```python
from build123d import *

# Parameters (mm, degrees)
SKETCH1_R           = 1.5
SKETCH1_R_2         = 1.35
SKETCH1_R_3         = 1.3
BOSS_EXTRUDE1_DEPTH = 3
BOSS_EXTRUDE2_START = 2
SKETCH2_W           = 64
SKETCH2_H           = 44
SKETCH2_R           = 1.3
BOSS_EXTRUDE2_DEPTH = 2
SKETCH3_W           = 64
SKETCH3_H           = 44
SKETCH3_W_2         = 60
SKETCH3_H_2         = 40
BOSS_EXTRUDE3_DEPTH = 12
SKETCH4_W           = 61
SKETCH4_H           = 41
SKETCH4_W_2         = 60
SKETCH4_H_2         = 40
CUT_EXTRUDE1_DEPTH  = 9
SKETCH5_R           = 3
CUT_EXTRUDE2_DEPTH  = 9
CUT_EXTRUDE3_START  = -9
CUT_EXTRUDE3_DEPTH  = 9
SKETCH7_W           = 66
SKETCH7_H           = 46
SKETCH7_W_2         = 64
SKETCH7_H_2         = 44
BOSS_EXTRUDE4_DEPTH = 14
SKETCH8_W           = 66
SKETCH8_H           = 46
BOSS_EXTRUDE5_DEPTH = 2
SKETCH9_R           = 6
SKETCH9_R_2         = 1.5
BOSS_EXTRUDE7_DEPTH = 4
FILLET1_R           = 5
FILLET2_R           = 2


with BuildPart() as part:
    # Sketch1 → Boss-Extrude1 (new body)
    # profile 1 of 12: a face of its own
    with BuildSketch(Plane.XY):
        with BuildLine():
            Line((-25.901923789, 20), (-28.5, 20))
            ThreePointArc((-28.5, 20), (-27.439339828, 19.560660172), (-27, 18.5))
            ThreePointArc((-27, 18.5), (-28.5, 17), (-30, 18.5))
            Line((-30, 18.5), (-30, 15.901923789))
            ThreePointArc((-30, 15.901923789), (-27, 15.901923789), (-25.5, 18.5))
            ThreePointArc((-25.5, 18.5), (-25.602222521, 19.276457135), (-25.901923789, 20))
        make_face()
    # profile 2 of 12: a face of its own
    with BuildSketch(Plane.XY):
        with BuildLine():
            Line((28.5, 20), (25.901923789, 20))
            ThreePointArc((25.901923789, 20), (26.378679656, 16.378679656), (30, 15.901923789))
            Line((30, 15.901923789), (30, 18.5))
            ThreePointArc((30, 18.5), (27.439339828, 17.439339828), (28.5, 20))
        make_face()
    # profile 3 of 12: a face of its own
    with BuildSketch(Plane.XY):
        with BuildLine():
            Line((30, -18.5), (30, -15.901923789))
            ThreePointArc((30, -15.901923789), (26.378679656, -16.378679656), (25.901923789, -20))
            Line((25.901923789, -20), (28.5, -20))
            ThreePointArc((28.5, -20), (27.439339828, -17.439339828), (30, -18.5))
        make_face()
    # profile 4 of 12: a face of its own
    with BuildSketch(Plane.XY):
        with BuildLine():
            ThreePointArc((-25.5, -18.5), (-27, -15.901923789), (-30, -15.901923789))
            Line((-30, -15.901923789), (-30, -18.5))
            ThreePointArc((-30, -18.5), (-28.5, -17), (-27, -18.5))
            ThreePointArc((-27, -18.5), (-27.439339828, -19.560660172), (-28.5, -20))
            Line((-28.5, -20), (-25.901923789, -20))
            ThreePointArc((-25.901923789, -20), (-25.602222521, -19.276457135), (-25.5, -18.5))
        make_face()
    # profile 5 of 12: a face of its own
    with BuildSketch(Plane.XY):
        with BuildLine():
            Line((-28.5, 20), (-30, 20))
            Line((-30, 20), (-30, 18.5))
            ThreePointArc((-30, 18.5), (-29.560660172, 19.560660172), (-28.5, 20))
        make_face()
    # profile 6 of 12: a face of its own
    with BuildSketch(Plane.XY):
        with Locations((-28.5, 18.5)):
            Circle(SKETCH1_R)
        with Locations((-28.5, 18.5)):
            Circle(SKETCH1_R_2, mode=Mode.SUBTRACT)
    # profile 7 of 12: a face of its own
    with BuildSketch(Plane.XY):
        with BuildLine():
            Line((30, 20), (28.5, 20))
            ThreePointArc((28.5, 20), (29.560660172, 19.560660172), (30, 18.5))
            Line((30, 18.5), (30, 20))
        make_face()
    # profile 8 of 12: a face of its own
    with BuildSketch(Plane.XY):
        with Locations((28.5, 18.5)):
            Circle(SKETCH1_R)
        with Locations((28.5, 18.5)):
            Circle(SKETCH1_R_3, mode=Mode.SUBTRACT)
    # profile 9 of 12: a face of its own
    with BuildSketch(Plane.XY):
        with BuildLine():
            Line((30, -20), (30, -18.5))
            ThreePointArc((30, -18.5), (29.560660172, -19.560660172), (28.5, -20))
            Line((28.5, -20), (30, -20))
        make_face()
    # profile 10 of 12: a face of its own
    with BuildSketch(Plane.XY):
        with Locations((28.5, -18.5)):
            Circle(SKETCH1_R)
        with Locations((28.5, -18.5)):
            Circle(SKETCH1_R_3, mode=Mode.SUBTRACT)
    # profile 11 of 12: a face of its own
    with BuildSketch(Plane.XY):
        with BuildLine():
            ThreePointArc((-28.5, -20), (-29.560660172, -19.560660172), (-30, -18.5))
            Line((-30, -18.5), (-30, -20))
            Line((-30, -20), (-28.5, -20))
        make_face()
    # profile 12 of 12: a face of its own
    with BuildSketch(Plane.XY):
        with Locations((-28.5, -18.5)):
            Circle(SKETCH1_R)
        with Locations((-28.5, -18.5)):
            Circle(SKETCH1_R_3, mode=Mode.SUBTRACT)
    extrude(amount=BOSS_EXTRUDE1_DEPTH)

    # Sketch2 → Boss-Extrude2 (add)
    # profile 1 of 4: a face of its own
    with BuildSketch(Plane(origin=(0, 0, 0), x_dir=(-1, 0, 0), z_dir=(0, 0, -1)).offset(BOSS_EXTRUDE2_START)):
        Rectangle(SKETCH2_W, SKETCH2_H)
        Polygon((-30, 15.901923789), (-30, 20), (-25.901923789, 20), (30, 20), (30, -20), (-30, -20), align=None, mode=Mode.SUBTRACT)
    # profile 2 of 4: a face of its own
    with BuildSketch(Plane(origin=(0, 0, 0), x_dir=(-1, 0, 0), z_dir=(0, 0, -1)).offset(BOSS_EXTRUDE2_START)):
        with BuildLine():
            Line((30, 20), (-25.901923789, 20))
            ThreePointArc((-25.901923789, 20), (-26.378679656, 16.378679656), (-30, 15.901923789))
            Line((-30, 15.901923789), (-30, -20))
            Line((-30, -20), (30, -20))
            Line((30, -20), (30, 20))
        make_face()
    # profile 3 of 4: a face of its own
    with BuildSketch(Plane(origin=(0, 0, 0), x_dir=(-1, 0, 0), z_dir=(0, 0, -1)).offset(BOSS_EXTRUDE2_START)):
        with BuildLine():
            ThreePointArc((-30, 15.901923789), (-26.378679656, 16.378679656), (-25.901923789, 20))
            Line((-25.901923789, 20), (-30, 20))
            Line((-30, 20), (-30, 15.901923789))
        make_face()
        with Locations(Location((-28.5, 18.5, 0), (0, 0, 180))):
            Circle(SKETCH2_R, mode=Mode.SUBTRACT)
    # profile 4 of 4: a face of its own
    with BuildSketch(Plane(origin=(0, 0, 0), x_dir=(-1, 0, 0), z_dir=(0, 0, -1)).offset(BOSS_EXTRUDE2_START)):
        with Locations(Location((-28.5, 18.5, 0), (0, 0, 180))):
            Circle(SKETCH2_R)
    extrude(amount=-BOSS_EXTRUDE2_DEPTH)

    # Sketch3 → Boss-Extrude3 (add)
    with BuildSketch(Plane.XY):
        Rectangle(SKETCH3_W, SKETCH3_H)
        Rectangle(SKETCH3_W_2, SKETCH3_H_2, mode=Mode.SUBTRACT)
    extrude(amount=BOSS_EXTRUDE3_DEPTH)

    # Sketch4 → Cut-Extrude1 (cut)
    with BuildSketch(Plane.XY.offset(12)):
        Rectangle(SKETCH4_W, SKETCH4_H)
        Rectangle(SKETCH4_W_2, SKETCH4_H_2, mode=Mode.SUBTRACT)
    extrude(amount=-CUT_EXTRUDE1_DEPTH, mode=Mode.SUBTRACT)

    # Sketch5 → Cut-Extrude2 (cut)
    with BuildSketch(Plane.XY.offset(3)):
        with Locations((28.5, -18.5)):
            Circle(SKETCH5_R)
        with Locations((-28.5, -18.5)):
            Circle(SKETCH5_R)
        with Locations((-28.5, 18.564453257)):
            Circle(SKETCH5_R)
        with Locations((28.5, 18.564453257)):
            Circle(SKETCH5_R)
    extrude(amount=CUT_EXTRUDE2_DEPTH, mode=Mode.SUBTRACT)

    # Sketch6 → Cut-Extrude3 (cut)
    with BuildSketch(Plane.XY.offset(CUT_EXTRUDE3_START)):
        with BuildLine():
            Line((30, -15.901923789), (30, 15.901923789))
            ThreePointArc((30, 15.901923789), (26.378679656, 16.378679656), (25.901923789, 20))
            Line((25.901923789, 20), (-25.901923789, 20))
            ThreePointArc((-25.901923789, 20), (-26.378679656, 16.378679656), (-30, 15.901923789))
            Line((-30, 15.901923789), (-30, -15.901923789))
            ThreePointArc((-30, -15.901923789), (-26.378679656, -16.378679656), (-25.901923789, -20))
            Line((-25.901923789, -20), (25.901923789, -20))
            ThreePointArc((25.901923789, -20), (26.378679656, -16.378679656), (30, -15.901923789))
        make_face()
    extrude(amount=CUT_EXTRUDE3_DEPTH, mode=Mode.SUBTRACT)

    # Sketch7 → Boss-Extrude4 (add)
    with BuildSketch(Plane(origin=(0, 0, -2), x_dir=(-1, 0, 0), z_dir=(0, 0, -1))):
        Rectangle(SKETCH7_W, SKETCH7_H)
        Rectangle(SKETCH7_W_2, SKETCH7_H_2, mode=Mode.SUBTRACT)
    extrude(amount=-BOSS_EXTRUDE4_DEPTH)

    # Sketch8 → Boss-Extrude5 (add)
    with BuildSketch(Plane(origin=(0, 0, -2), x_dir=(-1, 0, 0), z_dir=(0, 0, -1))):
        Rectangle(SKETCH8_W, SKETCH8_H)
    extrude(amount=BOSS_EXTRUDE5_DEPTH)

    # Sketch9 → Boss-Extrude7 (add)
    # profile 1 of 6: a face of its own
    with BuildSketch(Plane(origin=(0, 0, -4), x_dir=(-1, 0, 0), z_dir=(0, 0, -1))):
        with Locations((39, 0)):
            Circle(SKETCH9_R)
        with Locations((39, 0)):
            Circle(SKETCH9_R_2, mode=Mode.SUBTRACT)
    # profile 2 of 6: a face of its own
    with BuildSketch(Plane(origin=(0, 0, -4), x_dir=(-1, 0, 0), z_dir=(0, 0, -1))):
        with BuildLine():
            ThreePointArc((33, 1e-09), (34.757359313, 4.242640687), (39, 6))
            Line((39, 6), (33, 6))
            Line((33, 6), (33, 1e-09))
        make_face()
    # profile 3 of 6: a face of its own
    with BuildSketch(Plane(origin=(0, 0, -4), x_dir=(-1, 0, 0), z_dir=(0, 0, -1))):
        with BuildLine():
            ThreePointArc((39, -6), (34.757359313, -4.242640687), (33, 1e-09))
            Line((33, 1e-09), (33, -6))
            Line((33, -6), (39, -6))
        make_face()
    # profile 4 of 6: a face of its own
    with BuildSketch(Plane(origin=(0, 0, -4), x_dir=(-1, 0, 0), z_dir=(0, 0, -1))):
        with Locations((-39, 0)):
            Circle(SKETCH9_R)
        with Locations((-39, 0)):
            Circle(SKETCH9_R_2, mode=Mode.SUBTRACT)
    # profile 5 of 6: a face of its own
    with BuildSketch(Plane(origin=(0, 0, -4), x_dir=(-1, 0, 0), z_dir=(0, 0, -1))):
        with BuildLine():
            Line((-33, 0), (-33, 6))
            Line((-33, 6), (-39, 6))
            ThreePointArc((-39, 6), (-34.757359313, 4.242640687), (-33, 0))
        make_face()
    # profile 6 of 6: a face of its own
    with BuildSketch(Plane(origin=(0, 0, -4), x_dir=(-1, 0, 0), z_dir=(0, 0, -1))):
        with BuildLine():
            Line((-33, -6), (-33, 0))
            ThreePointArc((-33, 0), (-34.757359313, -4.242640687), (-39, -6))
            Line((-39, -6), (-33, -6))
        make_face()
    extrude(amount=-BOSS_EXTRUDE7_DEPTH)

    # Fillet1
    fillet1_edges = [part.edges().sort_by_distance(p)[0] for p in [
        (-33, 6, -2),
        (-33, -6, -2),
        (33, -6, -2),
        (33, 6, -2),
    ]]
    fillet(fillet1_edges, radius=FILLET1_R)

    # Fillet2
    fillet2_edges = [part.edges().sort_by_distance(p)[0] for p in [
        (-33, 23, 4),
        (33, -23, 4),
        (-33, -23, 4),
        (33, 23, 4),
    ]]
    fillet(fillet2_edges, radius=FILLET2_R)


solid = part.part
```
CAD build for the part. Positions are in the model's coordinates, mm. A direction names the side the tool comes from. Coordinates: 2 decimals unless noted, no trailing zeros. Order: outer loops, then holes, each group sorted by start corner. A loop starts at its lowest first (then second) coordinate and runs counter-clockwise, first axis right, second up. Notation, with made-up numbers: (56.5, 14) - (63.5, 14) arc R23 cw to (63.5, 34) - close; hole circle Ø1 at (-9.5, -38). An arc over 180 degrees is marked (long way). Answer in a Markdown table with one row per item.
1. Slice it at A-A, the plane x = -6. List the corners of the cut face in (y, z).
Answer:
| item | result |
|---|---|
| outline | (-23, -4) - (23, -4) - (23, 12) - (20.5, 12) - (20.5, 3) - (20, 3) - (20, -2) - (-20, -2) - (-20, 3) - (-20.5, 3) - (-20.5, 12) - (-23, 12) - close |
2. Pull direction X, two halves, no side cores. Call faces 1 (the face through (-29.8, -18.44, 1.48)), 2 (the face through (34, 8, -2)), 3 (the face through (-32.43, 22.4, 4.11)): +X half, -X half, draft (parallel to the pull), parting line (faces both ways), or undercut.
Answer:
| item | result |
|---|---|
| face 1 | undercut |
| face 2 | +X half |
| face 3 | -X half |
3. Drill centre lines: L1, parallel to Y at x = 28.5, z = 1.15; L2, parallel to Y at x = -19.5, z = 1.25; L3, parallel to X at y = 9.5, z = 1.5. Where is each one in solid material? Low to high. Write a range as from..to.
Answer:
| item | result |
|---|---|
| L1 | -23..-19.8, -17.2..-15.5, 15.5..17.2, 19.8..23 |
| L2 | -23..-20, 20..23 |
| L3 | -33..-30, 30..33 |
4. Slice it at D-D, the plane y = 14.5. List the corners of the cut face in (x, z), then the cut area to 3 significant figures.
Answer:
| item | result |
|---|---|
| outline | (-33, -4) - (33, -4) - (33, 12) - (30.5, 12) - (30.5, 3) - (30, 3) - (30, -2) - (-30, -2) - (-30, 3) - (-30.5, 3) - (-30.5, 12) - (-33, 12) - close |
| area | 207 mm² |
5. Flat gauge pins, fed straight in: P1, Ø2, axis at x = 28, y = 19, coming from the +Z side; P2, Ø2.5, axis at x = 28.5, y = 18.5, coming from the +Z side; P3, Ø2, axis at x = 1, y = 8.5, coming from the +Z side; P4, Ø4, axis at y = 0.5, z = 0.5, coming from the -X side. Where does each tip first touch, or does it go through?
Answer:
| item | result |
|---|---|
| P1 | z = 3 |
| P2 | z = 0 |
| P3 | z = -2 |
| P4 | x = -45 |
6. 3-axis set-ups, long thin cutter, end or side, ignore diameter. For faces 4 (the face through (0, 23, 4)), 5 (the face through (0, 20, 0)), 6 (the face through (-36, 0, 0)): which of +Z, -Z, +X, -X, +Y, -Y reach the whole face in a straight line?
Answer:
| item | result |
|---|---|
| face 4 | +Z, -Z, +X, -X, +Y |
| face 5 | +Z |
| face 6 | +Z, -X, +Y, -Y |
7. Slice it at B-B, the plane y = 0. List the corners of the cut face in (x, z), then the cut area to 3 significant figures.
Answer:
| item | result |
|---|---|
| outline | (-45, -4) - (-40.5, -4) - (-40.5, 0) - (-45, 0) - close; (-37.5, -4) - (37.5, -4) - (37.5, 0) - (33, 0) - (33, 12) - (30.5, 12) - (30.5, 3) - (30, 3) - (30, -2) - (-30, -2) - (-30, 3) - (-30.5, 3) - (-30.5, 12) - (-33, 12) - (-33, 0) - (-37.5, 0) - close; (40.5, -4) - (45, -4) - (45, 0) - (40.5, 0) - close |
| area | 279 mm² |
8. Slice it at C-C, the plane z = 10.5. List the corners of the cut face in (x, y), then the cut area to 3 significant figures.
Answer:
| item | result |
|---|---|
| outline | (-33, -21) arc R2 ccw to (-31, -23) - (31, -23) arc R2 ccw to (33, -21) - (33, 21) arc R2 ccw to (31, 23) - (-31, 23) arc R2 ccw to (-33, 21) - close; hole (-30.5, -16.26) arc R3 ccw (long way) to (-26.26, -20.5) - (26.26, -20.5) arc R3 ccw (long way) to (30.5, -16.26) - (30.5, 16.33) arc R3 ccw (long way) to (26.21, 20.5) - (-26.21, 20.5) arc R3 ccw (long way) to (-30.5, 16.33) - close |
| area | 506 mm² |
